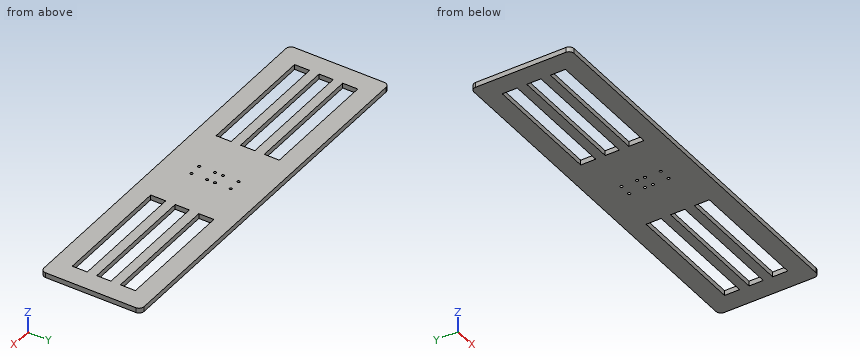
```python
from build123d import *

# Parameters (mm, degrees)
SKETCH1_W            = 482.6
SKETCH1_H            = 101.6
SKETCH1_W_2          = 152.4
SKETCH1_H_2          = 19.05
SKETCH1_H_3          = 18
BOSS_EXTRUDE1_DEPTH  = 6.35
M3_CLEARANCE_HOLE1_D = 3.4
SKETCH4_W            = 482.6
SKETCH4_H            = 12.7
BOSS_EXTRUDE2_DEPTH  = 6.35
FILLET2_R            = 6.35


with BuildPart() as part:
    # Sketch1 → Boss-Extrude1 (new body)
    with BuildSketch(Plane.XY):
        Rectangle(SKETCH1_W, SKETCH1_H)
        with Locations((-139.7, -30.525)):
            Rectangle(SKETCH1_W_2, SKETCH1_H_2, mode=Mode.SUBTRACT)
        with Locations((139.7, -30.525)):
            Rectangle(SKETCH1_W_2, SKETCH1_H_2, mode=Mode.SUBTRACT)
        with Locations((-139.7, 0)):
            Rectangle(SKETCH1_W_2, SKETCH1_H_3, mode=Mode.SUBTRACT)
        with Locations((-139.7, 30.525)):
            Rectangle(SKETCH1_W_2, SKETCH1_H_2, mode=Mode.SUBTRACT)
        with Locations((139.7, 0)):
            Rectangle(SKETCH1_W_2, SKETCH1_H_3, mode=Mode.SUBTRACT)
        with Locations((139.7, 30.525)):
            Rectangle(SKETCH1_W_2, SKETCH1_H_2, mode=Mode.SUBTRACT)
    extrude(amount=BOSS_EXTRUDE1_DEPTH)

    # M3 Clearance Hole1 (through all)
    with Locations(Plane.XY.offset(6.35)):
        with Locations((7.625, 5), (7.625, 25), (7.625, -5), (-7.625, 25), (-7.625, 5), (7.625, -25), (-7.625, -25), (-7.625, -5)):
            Hole(M3_CLEARANCE_HOLE1_D / 2)

    # Sketch4 → Boss-Extrude2 (add)
    with BuildSketch(Plane(origin=(0, 0, 0), x_dir=(-1, 0, 0), z_dir=(0, 0, -1))):
        with Locations((0, -57.15)):
            Rectangle(SKETCH4_W, SKETCH4_H)
        with Locations((0, 57.15)):
            Rectangle(SKETCH4_W, SKETCH4_H)
    extrude(amount=-BOSS_EXTRUDE2_DEPTH)

    # Fillet2
    fillet2_edges = [part.edges().sort_by_distance(p)[0] for p in [
        (241.3, -63.5, 3.175),
        (-241.3, -63.5, 3.175),
        (241.3, 63.5, 3.175),
        (-241.3, 63.5, 3.175),
    ]]
    fillet(fillet2_edges, radius=FILLET2_R)


solid = part.part
```
The model under review builds one solid part; all positions refer to its coordinate system, in mm. Give positions to 0.01 mm unless a question says otherwise; leave off trailing zeros. Order: outer loops, then holes, each group sorted by start corner. A loop starts at its lowest first (then second) coordinate and runs counter-clockwise, first axis right, second up. Notation, with made-up numbers: (4.5, 44) - (16.5, 44) arc R30 ccw to (16.5, 82) - close; hole circle Ø6 at (12, 81). An arc over 180 degrees is marked (long way). Use CSV: the item, a comma, the result in double quotes. Start each with the question number.
Q1. We need section B-B, the plane y = -34. Write out the cut boundary in (x, z).
Q2. To check wall thickness, follow line 1 along Y through (x, z) = (-86, 0.5); line 2 along X through (y, z) = (-39, 2.75); line 3 along X through (y, z) = (-3.5, 4.75) (3 decimals). State the ranges of each line that lie inside material, in increasing order. Write a range as [from, to].
Q3. We need section A-A, the plane x = -176.5. Write out the cut boundary in (y, z), and give its area (3 significant figures).
Q4. Clearance check with a flat-ended pin moving along its axis: pin 1 Ø3 at (x, y) = (7.625, 25) entering from +Z. State where the tip first meets the part, or that it passes through.
Q5. We need section C-C, the plane z = 3.5. State how many separate pieces and enclosed holes the cut face has, and give its area (3 significant figures).
Outcome:
1,outline,"(-241.3, 0) - (-215.9, 0) - (-215.9, 6.35) - (-241.3, 6.35) - close; (-63.5, 0) - (63.5, 0) - (63.5, 6.35) - (-63.5, 6.35) - close; (215.9, 0) - (241.3, 0) - (241.3, 6.35) - (215.9, 6.35) - close"
2,line 1,"y = [-63.5, -40.05], [-21, -9], [9, 21], [40.05, 63.5]"
2,line 2,"x = [-241.3, -215.9], [-63.5, 63.5], [215.9, 241.3]"
2,line 3,"x = [-241.3, -215.9], [-63.5, -8.425], [-6.825, 6.825], [8.425, 63.5], [215.9, 241.3]"
3,outline,"(-63.5, 0) - (-40.05, 0) - (-40.05, 6.35) - (-63.5, 6.35) - close; (-21, 0) - (-9, 0) - (-9, 6.35) - (-21, 6.35) - close; (9, 0) - (21, 0) - (21, 6.35) - (9, 6.35) - close; (40.05, 0) - (63.5, 0) - (63.5, 6.35) - (40.05, 6.35) - close"
3,area,"450 mm^2"
4,pin 1,"passes through"
5,separate pieces,"1"
5,enclosed holes,"14"
5,area,"44,100 mm^2"
